Check sheet for the modelled part. Datum: model origin and axes. Units: mm. A direction names the side the tool comes from. Coordinates: 2 decimals unless noted, no trailing zeros. Write each question's results on one line, items separated by ' | '. Start each with the question number.
1. Draft check along Y on faces 1 (the face through (-117.16, -106.65, 3.39)), 2 (the face through (-158.363, -10, 2)), 3 (the face through (-116, -108.159, 2)). Enter one of: released by +Y, released by -Y, zero draft, split by the parting line, or undercut.
2. Thickness scan on line 1 (Y direction, x = -113, z = 4.35); line 2 (Y direction, x = -88, z = 0.55); line 3 (X direction, y = -9.5, z = 3). Record the ranges inside material, lowest first. Write a range as [from, to].
3. Tool access check on faces 4 (the face through (-78.588, 58.554, 3.387)), 5 (the face through (-143.316, -103.876, 1.727)). Record the directions out of +Z, -Z, +X, -X, +Y, -Y that give a thin tool (end or side, any length) a straight path to the whole face; none if there is none.
4. Gauge pin test, flat ends, axial feed: P1, Ø2, axis at x = -88.36, y = -105.66, coming from the +Z side; P2, Ø4, axis at x = -88.36, y = -105.66, coming from the -Z side; P3, Ø1.8, axis at y = -58.16, z = 2.5, coming from the -X side. Record the tip position at first contact, or that the pin passes through.
```python
from build123d import *

# Parameters (mm, degrees)
SKETCH1_W                                           = 85
SKETCH1_H                                           = 200
BOSS_EXTRUDE1_DEPTH                                 = 5
CBORE_FOR_4_BINDING_HEAD_MACHINE_SCREW1_D           = 3.4544
CBORE_FOR_4_BINDING_HEAD_MACHINE_SCREW1_CBORE_D     = 6.74624
CBORE_FOR_4_BINDING_HEAD_MACHINE_SCREW1_CBORE_DEPTH = 1.7272
CBORE_FOR_4_BINDING_HEAD_MACHINE_SCREW2_D           = 3.2639
CBORE_FOR_4_BINDING_HEAD_MACHINE_SCREW2_DEPTH       = 5
CBORE_FOR_4_BINDING_HEAD_MACHINE_SCREW2_CBORE_D     = 6.74624
CBORE_FOR_4_BINDING_HEAD_MACHINE_SCREW2_CBORE_DEPTH = 1.7272
F_4_40_TAPPED_HOLE2_D                               = 2.2606
F_4_40_TAPPED_HOLE2_DEPTH                           = 7.6
F_4_40_TAPPED_HOLE2_TIP                             = 0.679152758
SKETCH10_R                                          = 4.5
CUT_EXTRUDE2_DEPTH                                  = 6
SKETCH10_6_R                                        = 6.35
CUT_EXTRUDE3_DEPTH                                  = 3


with BuildPart() as part:
    # Sketch1 → Boss-Extrude1 (new body)
    with BuildSketch(Plane.XY):
        with Locations((-115.863171355, -8.158567775)):
            Rectangle(SKETCH1_W, SKETCH1_H)
    extrude(amount=BOSS_EXTRUDE1_DEPTH)

    # CBORE for #4 Binding Head Machine Screw1 (through all)
    with Locations(Plane(origin=(0, 0, 0), x_dir=(-1, 0, 0), z_dir=(0, 0, -1))):
        with Locations((78.363171355, 56.841432225), (78.363171355, -8.158567775), (78.363171355, -73.158567775)):
            CounterBoreHole(CBORE_FOR_4_BINDING_HEAD_MACHINE_SCREW1_D / 2, CBORE_FOR_4_BINDING_HEAD_MACHINE_SCREW1_CBORE_D / 2, CBORE_FOR_4_BINDING_HEAD_MACHINE_SCREW1_CBORE_DEPTH)

    # CBORE for #4 Binding Head Machine Screw2
    with Locations(Plane(origin=(0, 0, 0), x_dir=(-1, 0, 0), z_dir=(0, 0, -1))):
        with Locations((88.363171355, 89.341432225), (115.863171355, 89.341432225), (143.363171355, 89.341432225), (143.363171355, -105.658567775), (115.863171355, -105.658567775), (88.363171355, -105.658567775)):
            CounterBoreHole(CBORE_FOR_4_BINDING_HEAD_MACHINE_SCREW2_D / 2, CBORE_FOR_4_BINDING_HEAD_MACHINE_SCREW2_CBORE_D / 2, CBORE_FOR_4_BINDING_HEAD_MACHINE_SCREW2_CBORE_DEPTH, depth=CBORE_FOR_4_BINDING_HEAD_MACHINE_SCREW2_DEPTH)

    # #4-40 Tapped Hole2
    with Locations(Plane.ZY.offset(158.363171355)):
        with Locations((2.5, -58.158567775), (2.5, 41.841432225)):
            Hole(F_4_40_TAPPED_HOLE2_D / 2, depth=F_4_40_TAPPED_HOLE2_DEPTH)
            with Locations((0, 0, -(F_4_40_TAPPED_HOLE2_DEPTH + F_4_40_TAPPED_HOLE2_TIP / 2))):  # 118° drill point
                Cone(0, F_4_40_TAPPED_HOLE2_D / 2, F_4_40_TAPPED_HOLE2_TIP, mode=Mode.SUBTRACT)

    # Sketch10 → Cut-Extrude2 (cut, through all)
    with BuildSketch(Plane(origin=(0, 0, 0), x_dir=(-1, 0, 0), z_dir=(0, 0, -1))):
        with Locations((113.363171355, -48.158567775)):
            Circle(SKETCH10_R)
    extrude(amount=-CUT_EXTRUDE2_DEPTH, mode=Mode.SUBTRACT)

    # Sketch10<6> → Cut-Extrude3 (cut)
    with BuildSketch(Plane(origin=(0, 0, 0), x_dir=(-1, 0, 0), z_dir=(0, 0, -1))):
        with Locations((113.363171355, -48.158567775)):
            Circle(SKETCH10_6_R)
    extrude(amount=-CUT_EXTRUDE3_DEPTH, mode=Mode.SUBTRACT)


solid = part.part
```
Established:
1) face 1: undercut | face 2: zero draft | face 3: released by -Y
2) line 1: [-108.16, -52.64], [-43.67, 91.84] | line 2: [-102.31, 85.99] | line 3: [-158.36, -79.45], [-77.28, -73.36]
3) face 4: +Z, -Z | face 5: -Z
4) P1: through | P2: z = 1.73 | P3: x = -150.63
